The listing builds one solid part. Answer for the finished solid, in the listing's coordinates (mm). A direction names the side the tool comes from. Coordinates: 2 decimals unless noted, no trailing zeros. Loops run counter-clockwise (first coordinate to the right, second up) from the corner with the lowest first, then second, coordinate; pieces in that order, holes last. Notation, with made-up numbers: M 5,76.25 L 22,76.25 A13 cw 22,95.25 Z; hole C 14,32 d10. An arc over 180 degrees is marked long. Answer in a Markdown table with one row per item. Add a question column.
from build123d import *

# Parameters (mm, degrees)
F1_DEPTH = 1400
F2_W     = 20
F2_H     = 100
F3_DEPTH = 5


with BuildPart() as f1:
    # F0 (on Front) → F1 (new body)
    with BuildSketch(Plane.XZ):
        with BuildLine():
            Line((49.962816, 35.773941), (-50.037184, 35.773941))
            Line((-50.037184, 35.773941), (-50.037184, -14.226059))
            Line((-50.037184, -14.226059), (-46.350433, -14.226059))
            ThreePointArc((-46.350433, -14.226059), (-43.590398, -13.121264), (-42.355, -10.417164))
            Line((-42.355, -10.417164), (-40.749153, 23.156153))
            ThreePointArc((-40.749153, 23.156153), (-38.227094, 28.613997), (-32.616079, 30.773941))
            Line((-32.616079, 30.773941), (32.683921, 30.773941))
            ThreePointArc((32.683921, 30.773941), (38.203989, 28.564351), (40.674785, 23.156153))
            Line((40.674785, 23.156153), (42.280633, -10.417164))
            ThreePointArc((42.280633, -10.417164), (43.516031, -13.121264), (46.276065, -14.226059))
            Line((46.276065, -14.226059), (49.962816, -14.226059))
            Line((49.962816, -14.226059), (49.962816, 35.773941))
        make_face()
    extrude(amount=-F1_DEPTH)

    # F2 (on face) → F3 (cut, through all)
    with BuildSketch(Plane.XY.offset(35.773941)):
        with Locations((0, 132)):
            Rectangle(F2_W, F2_H)
        with Locations((0, 1257)):
            Rectangle(F2_W, F2_H)
    extrude(amount=-F3_DEPTH, mode=Mode.SUBTRACT)


solid = f1.part
(1) Straight lines are drawn through the part: line 1 (X direction, y = 820, z = -8); line 2 (X direction, y = 201.5, z = -6); line 3 (Z direction, x = 46, y = 363.5). For each, find the intervals that lie inside material, in ascending order.
(2) The mould has two halves that part along X. Classify faces 3 (the face through (-4, 1400, 31)), 4 (the face through (41.466, 690.2, 6.605)), 5 (the face through (-50.037, 690, 11)), 6 (the face through (0, 690, 30.774)): released by +X, released by -X, zero draft, split by the parting line, or undercut.
(3) Each of these flat-tipped pins is pushed along its axis until it touches: pin 1 (1.5 mm diameter, centred on x = 35.5, y = 984.5, fed in from -Z); pin 2 (2 mm diameter, centred on x = 37.5, y = 318, fed in from -Z); pin 3 (4 mm diameter, centred on x = 28, y = 582.5, fed in from -Z). Where does it stop, or does it pass through?
(4) A cutting plane is placed at C-C (y = 647). Give the vertices of the cut face in (x, z) (3 decimals), plus the area to 3 significant figures.
(5) For faces 1 (the face through (-41.563, 690.2, 6.134)), 2 (the face through (1, 690, 35.774)), determine the directions among +Z, -Z, +X, -X, +Y, -Y from which every point of the face is accessible in a straight line to the end or side of a thin tool.
(6) A cutting plane is placed at B-B (z = 0.5). Give the vertices of the cut face in (x, y), plus the area to 3 significant figures.
(7) A cutting plane is placed at A-A (y = 1231.5). Give the vertices of the cut face in (x, z) (3 decimals).
Solved:
| question | item | result |
|---|---|---|
| 1 | line 1 | x = -50.04 to -42.24, 42.17 to 49.96 |
| 1 | line 2 | x = -50.04 to -42.14, 42.07 to 49.96 |
| 1 | line 3 | z = -14.22 to 35.77 |
| 2 | face 3 | zero draft |
| 2 | face 4 | undercut |
| 2 | face 5 | released by -X |
| 2 | face 6 | undercut |
| 3 | pin 1 | stops at z = 29.94 |
| 3 | pin 2 | stops at z = 28.27 |
| 3 | pin 3 | stops at z = 30.77 |
| 4 | outline | M -50.037,-14.226 L -46.35,-14.226 A4 ccw -42.355,-10.417 L -40.749,23.156 A8 cw -32.616,30.774 L 32.684,30.774 A8 cw 40.675,23.156 L 42.281,-10.417 A4 ccw 46.276,-14.226 L 49.963,-14.226 L 49.963,35.774 L -50.037,35.774 Z |
| 4 | area | 1,290 mm² |
| 5 | face 1 | -Z, +Y, -Y |
| 5 | face 2 | +Z, +X, -X, +Y, -Y |
| 6 | outline | M -50.04,0 L -41.83,0 L -41.83,1400 L -50.04,1400 Z; M 41.76,0 L 49.96,0 L 49.96,1400 L 41.76,1400 Z |
| 6 | area | 23,000 mm² |
| 7 | outline | M -50.037,-14.226 L -46.35,-14.226 A4 ccw -42.355,-10.417 L -40.749,23.156 A8 cw -32.616,30.774 L -10,30.774 L -10,35.774 L -50.037,35.774 Z; M 10,30.774 L 32.684,30.774 A8 cw 40.675,23.156 L 42.281,-10.417 A4 ccw 46.276,-14.226 L 49.963,-14.226 L 49.963,35.774 L 10,35.774 Z |
